```python
from build123d import *

# Parameters (mm, degrees)
SKETCH2_R      = 1.4478
EXTRUDE1_DEPTH = 4.9878


with BuildPart() as part:
    # Sketch1 → Revolve1 (revolve)
    with BuildSketch(Plane(origin=(0, 0, 0), x_dir=(0, 0, -1), z_dir=(1, 0, 0))):
        Polygon((0, 4.7371), (0, 0), (3.9878, 0), (3.9878, 4.0005), (1.3716, 4.0005), (1.3716, 3.7465), (0.8636, 3.7465), (0.8636, 4.7371), align=None)
    revolve(axis=Axis((0, 0, 0), (0, 0, -1)))

    # Sketch2 → Extrude1 (cut, through all)
    with BuildSketch(Plane.XY):
        Circle(SKETCH2_R)
    extrude(amount=-EXTRUDE1_DEPTH, mode=Mode.SUBTRACT)

    # Sketch3 → Cut-Revolve1 (revolve, cut)
    with BuildSketch(Plane(origin=(0, 0, 0), x_dir=(0, 0, -1), z_dir=(1, 0, 0))):
        Polygon((3.9878, 1.9558), (3.7338, 1.9558), (3.7338, 2.9845), (3.9878, 3.4925), align=None)
        Polygon((0, 1.9558), (0.254, 1.9558), (0.254, 3.032275316), (0.508, 3.032275316), (0.508, 3.4671), (0, 3.4671), align=None)
    revolve(axis=Axis((0, 0, 0), (0, 0, -1)), mode=Mode.SUBTRACT)


solid = part.part
```
CAD build for the part. Positions are in the model's coordinates, mm. A direction names the side the tool comes from. Coordinates: 2 decimals unless noted, no trailing zeros. Order: outer loops, then holes, each group sorted by start corner. A loop starts at its lowest first (then second) coordinate and runs counter-clockwise, first axis right, second up. Notation, with made-up numbers: (-38, 80) - (-24, 80) arc R29 ccw to (-24, 106) - close; hole circle Ø8 at (72, -0.75). An arc over 180 degrees is marked (long way). Use a Markdown table: item, result. Add a question column.
(1) Which spindle directions (+Z, -Z, +X, -X, +Y, -Y) get a long thin tool onto all of the face, cutting with end or side? Do faces 5 (the face through (2.9, 1.9, -0.3)), 6 (the face through (-3.9, -0.9, -2.7)), 7 (the face through (-1, 4, -0.864)), 8 (the face through (-4.624, -1.027, -0.426)). Say none if no direction does.
(2) Drill centre lines: line 1 along Z through (x, y) = (4, -1.5); line 2 along Y through (x, z) = (-0.75, -2.9); line 3 along X through (y, z) = (-0.5, -2.4). Where is each one in solid material? Low to high. Write a range as [from, to].
(3) Flat gauge pin, fed straight in: pin 1 (2.5 mm diameter, centred on x = 0, y = 0, fed in from -Z). Where does the tip first touch, or does it go through?
(4) Saw through at A-A (z = -1.95). Give the cut face in (x, y), then the cut area to 3 significant figures.
(5) Pull direction Z, two halves, no side cores. Call faces 1 (the face through (-2, -1, -3.734)), 2 (the face through (-2, -1, -0.254)), 3 (the face through (3.715, -0.488, -1.114)), 4 (the face through (-0.314, -1.413, -1.966)): +Z half, -Z half, draft (parallel to the pull), parting line (faces both ways), or undercut.
(6) Saw through at B-B (z = -1.1). Give the cut face in (x, y), then the cut area to 3 significant figures.
Solved:
| question | item | result |
|---|---|---|
| 1 | face 5 | +Z |
| 1 | face 6 | -Z |
| 1 | face 7 | none |
| 1 | face 8 | +Z, -Z |
| 2 | line 1 | z = [-0.86, 0] |
| 2 | line 2 | y = [-3.93, -1.24], [1.24, 3.93] |
| 2 | line 3 | x = [-3.97, -1.36], [1.36, 3.97] |
| 3 | pin 1 | passes through |
| 4 | outline | circle Ø8 at (0, 0); hole circle Ø2.9 at (0, 0) |
| 4 | area | 43.7 mm² |
| 5 | face 1 | -Z half |
| 5 | face 2 | +Z half |
| 5 | face 3 | undercut |
| 5 | face 4 | draft |
| 6 | outline | circle Ø7.49 at (0, 0); hole circle Ø2.9 at (0, 0) |
| 6 | area | 37.5 mm² |
